```python
from build123d import *

# Parameters (mm, degrees)
SKETCH1_W           = 30
SKETCH1_H           = 111
BOSS_EXTRUDE1_DEPTH = 35
CUT_EXTRUDE1_DEPTH  = 118.456302638
SKETCH3_R           = 5
BOSS_EXTRUDE2_DEPTH = 10


with BuildPart() as part:
    # Sketch1 → Boss-Extrude1 (new body)
    with BuildSketch(Plane.XY):
        with Locations((0.810851631, 0)):
            Rectangle(SKETCH1_W, SKETCH1_H)
    extrude(amount=BOSS_EXTRUDE1_DEPTH)

    # Sketch2 → Cut-Extrude1 (cut, through all)
    with BuildSketch(Plane(origin=(0, 55.5, 0), x_dir=(1, 0, 0), z_dir=(0, 1, 0))):
        Polygon((5.810851631, -35), (15.810851631, -25), (15.810851631, -35), align=None)
        with BuildLine():
            Line((15.810851631, -7), (15.810851631, -17))
            ThreePointArc((15.810851631, -17), (10.810851631, -12), (15.810851631, -7))
        make_face()
        Polygon((-14.189148369, -25), (-14.189148369, -35), (-4.189148369, -35), align=None)
        with BuildLine():
            Line((-14.189148369, -7), (-14.189148369, -17))
            ThreePointArc((-14.189148369, -17), (-9.189148369, -12), (-14.189148369, -7))
        make_face()
    extrude(amount=-CUT_EXTRUDE1_DEPTH, mode=Mode.SUBTRACT)

    # Sketch3 → Boss-Extrude2 (add)
    with BuildSketch(Plane(origin=(0, 0, 0), x_dir=(-1, 0, 0), z_dir=(0, 0, -1))):
        with Locations(Location((0, 45.5, 0), (0, 0, 180))):
            Circle(SKETCH3_R)
        with Locations(Location((0, -45.5, 0), (0, 0, 180))):
            Circle(SKETCH3_R)
    extrude(amount=BOSS_EXTRUDE2_DEPTH)


solid = part.part
```
Geometry check sheet. Reference: the model listing, model coordinates, mm. A direction names the side the tool comes from. Coordinates: 2 decimals unless noted, no trailing zeros. Write each loop counter-clockwise with the first axis right and the second up, starting at its lowest first coordinate (ties: lowest second). Pieces come first, ordered by that corner, then holes. Notation, with made-up numbers: M 83,37 L 141,37 A30 cw 141,75 Z; hole C -3,26 d3. An arc over 180 degrees is marked long. Use one line per item in the form item = value. Start each with the question number.
1) Section check D-D on z = 12. Enter the section's corners in (x, y).
2) Release check for a two-part mould opening along Y. For faces 1 (the flat face through (0, -46, -10)), 2 (the cylindrical face through (-0.651, 40.543, -4.93)), 3 (the flat face through (1, -55.5, 17)) record: pulls with the +Y half, pulls with the -Y half, needs draft (parallel to the pull), parting line crosses it, or undercut.
3) Set-up check for faces 4 (the flat face through (15.811, -1, 21)), 5 (the cylindrical face through (-0.651, -50.457, -4.93)): record each of +Z, -Z, +X, -X, +Y, -Y from which the full face is reachable in a straight line by a thin tool's end or side.
4) Section check B-B on x = -3. Enter the section's corners in (y, z).
5) Thickness scan on probe 1 along Z at (x, y) = (0.5, 23.5); probe 2 along Z at (x, y) = (-10.5, 25.5); probe 3 along Z at (x, y) = (12, 18.5). Record the ranges inside material, lowest first. Write a range as from..to.
6) Go/stop test with a flat-tipped pin: pin 1 Ø2 at (y, z) = (-39, -4.5) entering from +X. Record where the tip stops, or that it passes through.
7) Section check A-A on y = 5.5. Enter the section's corners in (x, z).
8) Section check C-C on z = -1.5. Enter the section's corners in (x, y), and give its area (3 significant figures).
Responses:
q1.outline = M -9.19,-55.5 L 10.81,-55.5 L 10.81,55.5 L -9.19,55.5 Z
q2.face_1 = needs draft
q2.face_2 = undercut
q2.face_3 = pulls with the -Y half
q3.face_4 = +Z, -Z, +X, +Y, -Y
q3.face_5 = -Z
q4.outline = M -55.5,0 L -49.5,0 L -49.5,-10 L -41.5,-10 L -41.5,0 L 41.5,0 L 41.5,-10 L 49.5,-10 L 49.5,0 L 55.5,0 L 55.5,35 L -55.5,35 Z
q5.probe_1 = 0..35
q5.probe_2 = 0..8.63, 15.37..28.69
q5.probe_3 = 0..8.76, 15.24..28.81
q6.pin_1 = through
q7.outline = M -14.19,0 L 15.81,0 L 15.81,7 A5 cw 15.81,17 L 15.81,25 L 5.81,35 L -4.19,35 L -14.19,25 L -14.19,17 A5 cw -14.19,7 Z
q8.outline = C 0,-45.5 d10; C 0,45.5 d10
q8.area = 157 mm2
